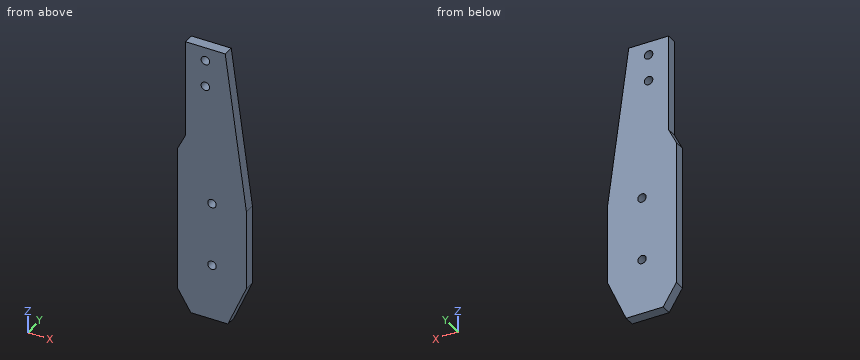
from build123d import *

# Parameters (mm, degrees)
BOSS_EXTRUDE1_DEPTH = 4
SKETCH2_R           = 1.6
CUT_EXTRUDE1_DEPTH  = 101.503731274


with BuildPart() as part:
    # Sketch1 → Boss-Extrude1 (new body)
    with BuildSketch(Plane(origin=(0, 0, 0), x_dir=(1, 0, 0), z_dir=(0, 1, 0))):
        Polygon((0, 0), (0, -54.5), (3, -60.5), (3, -97), (18, -97), (26, -38), (26, -8), (19, 8), (5, 8), align=None)
    extrude(amount=BOSS_EXTRUDE1_DEPTH)

    # Sketch2 → Cut-Extrude1 (cut, through all)
    with BuildSketch(Plane(origin=(0, 4, 0), x_dir=(1, 0, 0), z_dir=(0, 1, 0))):
        with Locations(Location((13, -13, 0), (0, 0, 270))):
            Circle(SKETCH2_R)
        with Locations(Location((13, -37, 0), (0, 0, 270))):
            Circle(SKETCH2_R)
        with Locations(Location((10.5, -82, 0), (0, 0, 270))):
            Circle(SKETCH2_R)
        with Locations(Location((10.5, -92, 0), (0, 0, 270))):
            Circle(SKETCH2_R)
    extrude(amount=-CUT_EXTRUDE1_DEPTH, mode=Mode.SUBTRACT)


solid = part.part
Work out the finished part from the listing and answer in its coordinate system (mm). Give positions to 0.01 mm unless a question says otherwise; leave off trailing zeros. Order: outer loops, then holes, each group sorted by start corner. A loop starts at its lowest first (then second) coordinate and runs counter-clockwise, first axis right, second up. Notation, with made-up numbers: (-39, 11.5) -> (16, 11.5) arc R24 cw to (16, 35.5) -> close; hole circle Ø3 at (-14.75, 47.25). An arc over 180 degrees is marked (long way). Answer as a JSON object with one key per item and string values. Group by question number.
1. Section D-D on z = 66.5 is taken. Determine the outline of the cut face in (x, y), plus the area to 3 significant figures.
2. Consider line 1 along X through (y, z) = (1.9, 37); line 2 along Z through (x, y) = (14, 1.9); line 3 along Z through (x, y) = (10.25, 3.25). Determine where each line is inside the solid, lowest interval first. Write a range as [from, to].
3. Section C-C on z = 82 is taken. Determine the outline of the cut face in (x, y).
4. Section B-B on y = 2.35 is taken. Determine the outline of the cut face in (x, z).
5. Flat-ended cylindrical pins translate along their axes: pin 1 Ø2 at (y, z) = (2.5, 72.5) entering from -X; pin 2 Ø1 at (y, z) = (1, 69) entering from +X; pin 3 Ø2.5 at (x, z) = (13, 37) entering from +Y; pin 4 Ø1 at (y, z) = (3, 80) entering from +X. Find the tip coordinate at first contact, or state that the pin passes through.
6. Section A-A on x = 13 is taken. Determine the outline of the cut face in (y, z).
Result sheet:
{
 "1": {"outline": "(3, 0) -> (22.14, 0) -> (22.14, 4) -> (3, 4) -> close", "area": "76.5 mm^2"},
 "2": {"line 1": "x = [0, 11.4], [14.6, 26]", "line 2": "z = [-8, 11.75], [14.25, 35.75], [38.25, 97]", "line 3": "z = [-8, 80.42], [83.58, 90.42], [93.58, 97]"},
 "3": {"outline": "(3, 0) -> (8.9, 0) -> (8.9, 4) -> (3, 4) -> close; (12.1, 0) -> (20.03, 0) -> (20.03, 4) -> (12.1, 4) -> close"},
 "4": {"outline": "(0, 0) -> (5, -8) -> (19, -8) -> (26, 8) -> (26, 38) -> (18, 97) -> (3, 97) -> (3, 60.5) -> (0, 54.5) -> close; hole circle Ø3.2 at (10.5, 82); hole circle Ø3.2 at (10.5, 92); hole circle Ø3.2 at (13, 13); hole circle Ø3.2 at (13, 37)"},
 "5": {"pin 1": "stops at x = 3", "pin 2": "stops at x = 21.86", "pin 3": "passes through", "pin 4": "stops at x = 20.37"},
 "6": {"outline": "(0, -8) -> (4, -8) -> (4, 11.4) -> (0, 11.4) -> close; (0, 14.6) -> (4, 14.6) -> (4, 35.4) -> (0, 35.4) -> close; (0, 38.6) -> (4, 38.6) -> (4, 97) -> (0, 97) -> close"}
}
